from build123d import *

# Parameters (mm, degrees)
BOSS_EXTRUDE2_DEPTH     = 60
CUT_EXTRUDE1_DEPTH      = 136.661343057
SKETCH3_R               = 12.5
BOSS_EXTRUDE3_DEPTH     = 80
SKETCH3_3_R             = 20
SKETCH3_3_R_2           = 12.5
BOSS_EXTRUDE4_DEPTH     = 25
FILLET2_R               = 6
CHAMFER1_SIZE           = 3
CUT_EXTRUDE2_DEPTH      = 136.661343057
CUT_EXTRUDE2_DEPTH_BACK = 136.661343057
SKETCH4_R               = 5


with BuildPart() as part:
    # Sketch1 → Boss-Extrude2 (new body)
    with BuildSketch(Plane(origin=(0, 0, 0), x_dir=(1, 0, 0), z_dir=(0, 1, 0))):
        Polygon((110, 10), (110, 0), (0, 0), (0, 52), (110, 52), (110, 42), (15, 42), (15, 10), align=None)
    extrude(amount=BOSS_EXTRUDE2_DEPTH)

    # Sketch2 → Cut-Extrude1 (cut, through all)
    with BuildSketch(Plane.XY):
        with BuildLine():
            Line((110, 60), (80, 60))
            ThreePointArc((80, 60), (101.213203436, 51.213203436), (110, 30))
            Line((110, 30), (110, 60))
        make_face()
        with BuildLine():
            Line((110, 0), (110, 30))
            ThreePointArc((110, 30), (101.213203436, 8.786796564), (80, 0))
            Line((80, 0), (110, 0))
        make_face()
    extrude(amount=-CUT_EXTRUDE1_DEPTH, mode=Mode.SUBTRACT)

    # Sketch3 → Boss-Extrude3 (add)
    with BuildSketch(Plane.ZY):
        with Locations((-26, 30)):
            Circle(SKETCH3_R)
    extrude(amount=BOSS_EXTRUDE3_DEPTH)

    # Sketch3<3> → Boss-Extrude4 (add)
    with BuildSketch(Plane.ZY):
        with Locations(Location((-26, 30, 0), (0, 0, 180))):
            Circle(SKETCH3_3_R)
        with Locations((-26, 30)):
            Circle(SKETCH3_3_R_2, mode=Mode.SUBTRACT)
    extrude(amount=BOSS_EXTRUDE4_DEPTH)

    # Fillet2
    fillet2_edges = [part.edges().sort_by_distance(p)[0] for p in [
        (0, 30, -6),
    ]]
    fillet(fillet2_edges, radius=FILLET2_R - 0.0001)  # a hair under: the kernel refuses the full size

    # Chamfer1
    chamfer1_edges = [part.edges().sort_by_distance(p)[0] for p in [
        (-80, 30, -38.5),
    ]]
    chamfer(chamfer1_edges, length=CHAMFER1_SIZE)

    # Sketch4 → Cut-Extrude2 (cut, two sides: drawn at the far end of the back side and taken through both)
    with BuildSketch(Plane.XY.offset(-CUT_EXTRUDE2_DEPTH_BACK)):
        with Locations((62, 30)):
            Circle(SKETCH4_R)
        with Locations((94, 30)):
            Circle(SKETCH4_R)
    extrude(amount=CUT_EXTRUDE2_DEPTH + CUT_EXTRUDE2_DEPTH_BACK, mode=Mode.SUBTRACT)


solid = part.part
Verification items for the finished model (mm, model axes). A direction names the side the tool comes from. Give positions to 0.01 mm unless a question says otherwise; leave off trailing zeros. Write each loop counter-clockwise with the first axis right and the second up, starting at its lowest first coordinate (ties: lowest second). Pieces come first, ordered by that corner, then holes.
(1) Cross-section at D-D (x = -58.5). Enter the section's corners in (y, z).
(2) Cross-section at A-A (x = 62). Enter the section's corners in (y, z), plus the area to 3 significant figures.
(3) Cross-section at B-B (z = -26). Enter the section's corners in (x, y), plus the area to 3 significant figures.
(4) Mould release check, pull along Z, two halves, no side actions. Record for faces 4 (the face through (15, 30, -26)), 5 (the face through (58, 27, -47)), 6 (the face through (56, 30, 0)): +Z half, -Z half, draft (parallel to the pull), parting line (faces both ways), or undercut.
(5) Access from +Z, -Z, +X, -X, +Y, -Y to the whole of each face (thin tool, end or side, straight path). Record for faces 1 (the face through (53, 30, -42)), 2 (the face through (32, 60, -9)), 3 (the face through (-50.64, 38.45, -35.21)).
(6) Gauge pin test, flat ends, axial feed: pin 1 (5 mm diameter, centred on x = -17, y = 27.5, fed in from +Z); pin 2 (10 mm diameter, centred on x = -16.5, z = -9.5, fed in from +Y); pin 3 (8 mm diameter, centred on x = -42, z = -39.5, fed in from +Y). Record the tip position at first contact, or that the pin passes through.
(7) Cross-section at C-C (x = 94). Enter the section's corners in (y, z).
(8) Material ranges on line 1 (Y direction, x = 62, z = -45.25); line 2 (Z direction, x = 75, y = 53.5); line 3 (X direction, y = 30, z = -2.5), recorded low to high.
Worked out:
1. outline: circle Ø25 at (30, -26)
2. outline: (0, -52) - (25, -52) - (25, -42) - (0, -42) - close; (0, -10) - (25, -10) - (25, 0) - (0, 0) - close; (35, -52) - (60, -52) - (60, -42) - (35, -42) - close; (35, -10) - (60, -10) - (60, 0) - (35, 0) - close
2. area: 1,000 mm2
3. outline: (-80, 20.5) - (-77, 17.5) - (-25, 17.5) - (-25, 10) - (-6, 10) arc R6 cw to (0, 4) - (0, 0) - (15, 0) - (15, 60) - (0, 60) - (0, 56) arc R6 cw to (-6, 50) - (-25, 50) - (-25, 42.5) - (-77, 42.5) - (-80, 39.5) - close
3. area: 3,280 mm2
4. face 4: undercut
4. face 5: draft
4. face 6: +Z half
5. face 1: +X, +Y, -Y
5. face 2: +Z, -Z, +X, -X, +Y
5. face 3: -X
6. pin 1: stops at z = -6
6. pin 2: stops at y = 46.36
6. pin 3: stops at y = 38.12
7. outline: (3.47, -52) - (25, -52) - (25, -42) - (3.47, -42) - close; (3.47, -10) - (25, -10) - (25, 0) - (3.47, 0) - close; (35, -52) - (56.53, -52) - (56.53, -42) - (35, -42) - close; (35, -10) - (56.53, -10) - (56.53, 0) - (35, 0) - close
8. line 1: y = 0 to 25, 35 to 60
8. line 2: z = -52 to -42, -10 to 0
8. line 3: x = -0.55 to 57, 67 to 89, 99 to 110
